Verification items for this drawing (mm, ordinates from the low corner). Coordinates: 2 decimals unless noted, no trailing zeros. Order: outer loops, then holes, each group sorted by start corner. A loop starts at its lowest first (then second) coordinate and runs counter-clockwise, first axis right, second up. Notation, with made-up numbers: (57.25, -12.75) -> (85.25, -12.75) arc R30 cw to (85.25, 25.25) -> close; hole circle Ø11 at (20, 27). An arc over 180 degrees is marked (long way). Write each question's results on one line, items separated by ' | '. Start each with the question number.
(1) Go/stop test with a flat-tipped pin: pin 1 (1.5 mm diameter, centred on x = 7.5, y = 2.5, fed in from -Z). Record where the tip stops, or that it passes through.
(2) Thickness scan on probe 1 along X at (y, z) = (3.4, 55); probe 2 along X at (y, z) = (0.7, 170). Record the ranges inside material, lowest first. Write a range as [from, to].
(3) Cross-section at A-A on z = 165. Enter the section's corners in (x, y).
(4) Cross-section at B-B on y = 3.35. Give the number of separate pieces and of enclosed holes in the cut face, and give its area (3 significant figures).
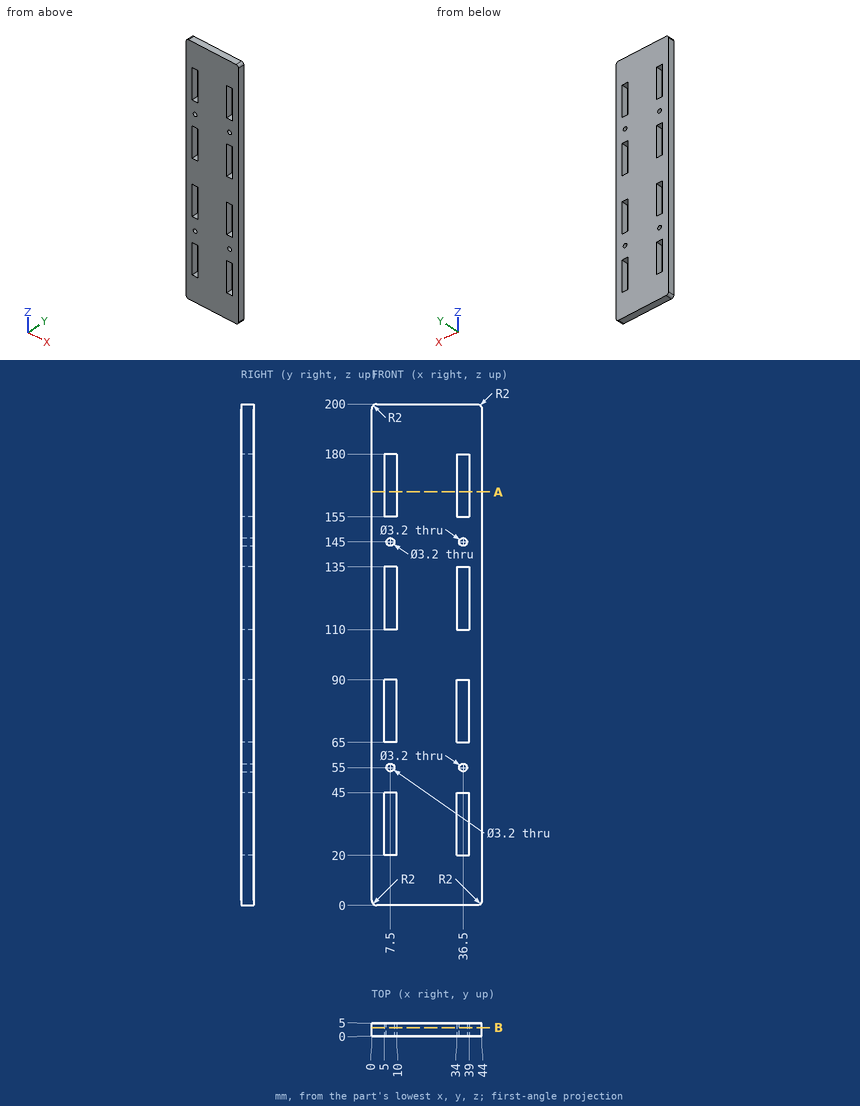
Results are:
1) pin 1: stops at z = 0
2) probe 1: x = [0, 5.9], [9.1, 34.9], [38.1, 44] | probe 2: x = [0, 5], [10, 34], [39, 44]
3) outline: (0, 0) -> (5, 0) -> (5, 5) -> (0, 5) -> close; (10, 0) -> (34, 0) -> (34, 5) -> (10, 5) -> close; (39, 0) -> (44, 0) -> (44, 5) -> (39, 5) -> close
4) separate pieces: 1 | enclosed holes: 12 | area: 7,760 mm2
